Can you work these out from the model? Positions are in its coordinate system, mm. Face numbers are marked on the shaded views. Coordinates: 2 decimals unless noted, no trailing zeros. Loops run counter-clockwise (first coordinate to the right, second up) from the corner with the lowest first, then second, coordinate; pieces in that order, holes last. Notation, with made-up numbers: (80.25, 20) -> (124.25, 20) arc R26 cw to (124.25, 38) -> close; hole circle Ø1 at (84.5, -20). An arc over 180 degrees is marked (long way). Use one line per item in the form item = value. Start each with the question number.
(1) Imagine slicing it at C-C (y = 5.25). List the corners of the cut face in (x, z) for me (3 decimals).
(2) Imagine slicing it at D-D (x = 0). List the corners of the cut face in (y, z) for me (3 decimals), plus the area to 3 significant figures.
(3) I'm going to push flat-ended pins straight in: pin 1 (7.5 mm diameter, centred on x = 8.128, y = 6.858, fed in from -Z); pin 2 (6 mm diameter, centred on x = -9.5, y = 5.5, fed in from +Z). Where does each tip first touch, or does it pass through?
(4) Imagine slicing it at B-B (x = -10.5). List the corners of the cut face in (y, z) for me.
(5) I need wall thicknesses on line 1 (Y direction, x = 0, z = 7); line 2 (X direction, y = 4.5, z = 3) (3 decimals); line 3 (Y direction, x = 0, z = 8.15) (3 decimals). Which ranges of each line are inside material? Lowest first, please. Write a range as [from, to].
(6) Imagine slicing it at A-A (y = -8.89). List the corners of the cut face in (x, z) for me (3 decimals), plus the area to 3 significant figures.
(7) Thinking about a two-plate mould opening in Y: for the marked faces 1, 2 and 3, which applies, released by +Y, released by -Y, zero draft, split by the parting line, or undercut?
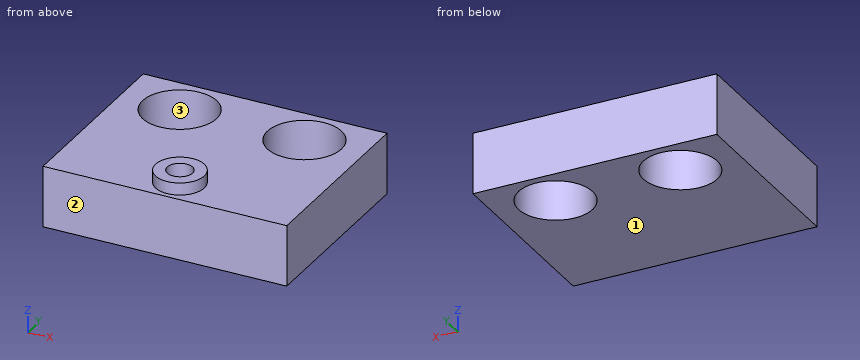
```python
from build123d import *

# Parameters (mm, degrees)
F0_W     = 31.75
F0_H     = 25.4
F0_R     = 4.826
F1_DEPTH = 7.9502
F2_R     = 3.175
F3_DEPTH = 1.5875
F4_R     = 1.651
F5_DEPTH = 4.7625


with BuildPart() as f1:
    # F0 (on Top) → F1 (new body)
    with BuildSketch(Plane.XY):
        Rectangle(F0_W, F0_H)
        with Locations((-8.128, 6.858)):
            Circle(F0_R, mode=Mode.SUBTRACT)
        with Locations((8.128, 6.858)):
            Circle(F0_R, mode=Mode.SUBTRACT)
    extrude(amount=F1_DEPTH)

    # F2 (on face) → F3 (join)
    with BuildSketch(Plane.XY.offset(7.9502)):
        with Locations((0, -8.89)):
            Circle(F2_R)
    extrude(amount=F3_DEPTH)

    # F4 (on face) → F5 (cut)
    with BuildSketch(Plane.XY.offset(9.5377)):
        with Locations((0, -8.89)):
            Circle(F4_R)
    extrude(amount=-F5_DEPTH, mode=Mode.SUBTRACT)


solid = f1.part
```
Worked out:
q1.outline = (-15.875, 0) -> (-12.678, 0) -> (-12.678, 7.95) -> (-15.875, 7.95) -> close; (-3.578, 0) -> (3.578, 0) -> (3.578, 7.95) -> (-3.578, 7.95) -> close; (12.678, 0) -> (15.875, 0) -> (15.875, 7.95) -> (12.678, 7.95) -> close
q2.outline = (-12.7, 0) -> (12.7, 0) -> (12.7, 7.95) -> (-5.715, 7.95) -> (-5.715, 9.538) -> (-7.239, 9.538) -> (-7.239, 4.775) -> (-10.541, 4.775) -> (-10.541, 9.538) -> (-12.065, 9.538) -> (-12.065, 7.95) -> (-12.7, 7.95) -> close
q2.area = 196 mm2
q3.pin_1 = through
q3.pin_2 = 7.95
q4.outline = (-12.7, 0) -> (2.66, 0) -> (2.66, 7.95) -> (-12.7, 7.95) -> close; (11.06, 0) -> (12.7, 0) -> (12.7, 7.95) -> (11.06, 7.95) -> close
q5.line_1 = [-12.7, -10.54], [-7.24, 12.7]
q5.line_2 = [-15.875, -12.339], [-3.917, 3.917], [12.339, 15.875]
q5.line_3 = [-12.065, -10.541], [-7.239, -5.715]
q6.outline = (-15.875, 0) -> (15.875, 0) -> (15.875, 7.95) -> (3.175, 7.95) -> (3.175, 9.538) -> (1.651, 9.538) -> (1.651, 4.775) -> (-1.651, 4.775) -> (-1.651, 9.538) -> (-3.175, 9.538) -> (-3.175, 7.95) -> (-15.875, 7.95) -> close
q6.area = 247 mm2
q7.face_1 = zero draft
q7.face_2 = released by -Y
q7.face_3 = undercut
